Job drawing, mm, ordinate dimensions from the low corner. One solid piece. Round coordinates to 2 decimals unless told otherwise and drop trailing zeros. Write each loop counter-clockwise with the first axis right and the second up, starting at its lowest first coordinate (ties: lowest second). Pieces come first, ordered by that corner, then holes.
1) Flat gauge pin, fed straight in: pin 1 (4 mm diameter, centred on x = 20, z = 6, fed in from +Y) (1 decimal). Where does the tip first touch, or does it go through?
2) Saw through at A-A on z = 11.75. Write the cut outline in (x, y) (1 decimal), and give its area (3 significant figures).
3) Drill centre lines: L1, parallel to Y at x = 5, z = 10.5 (1 decimal); L2, parallel to Y at x = 9.5, z = 20; L3, parallel to X at y = 21.75, z = 11.75 (1 decimal). Where is each one in solid material? Low to high.
4) Saw through at B-B on x = 34. Write the cut outline in (y, z) (1 decimal).
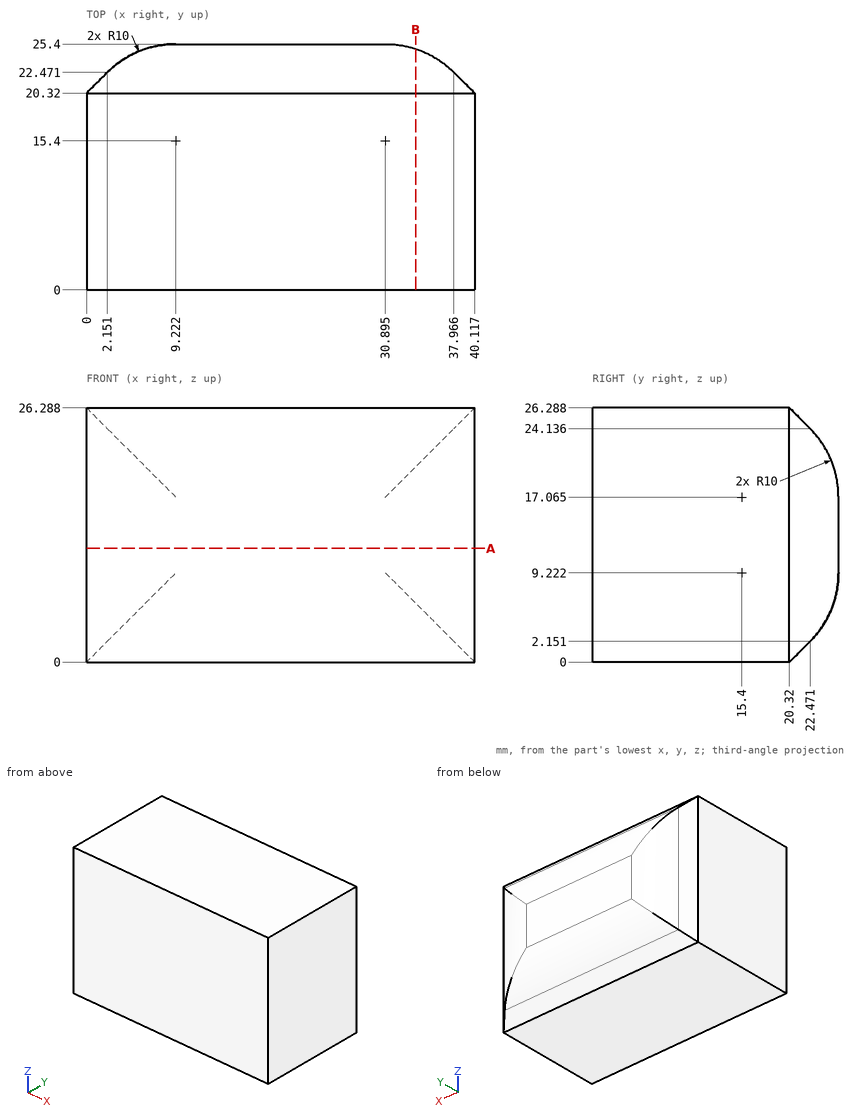
Completed:
1. pin 1: stops at y = 25.3
2. outline: (0, 0) - (40.1, 0) - (40.1, 20.3) - (38, 22.5) arc R10 ccw to (30.9, 25.4) - (9.2, 25.4) arc R10 ccw to (2.2, 22.5) - (0, 20.3) - close
2. area: 989 mm2
3. L1: y = 0 to 24.5
3. L2: y = 0 to 24.96
3. L3: x = 1.4 to 38.7
4. outline: (0, 0) - (20.3, 0) - (22.5, 2.2) arc R10 ccw to (24.9, 6.1) - (24.9, 20.2) arc R10 ccw to (22.5, 24.1) - (20.3, 26.3) - (0, 26.3) - close
